```python
from build123d import *

# Parameters (mm, degrees)
ESQUISSE6_W                  = 10
ESQUISSE6_H                  = 1
ENL_V_MAT_EXTRU_3_DEPTH      = 4
ENL_V_MAT_EXTRU_3_DEPTH_BACK = 4


with BuildPart() as part:
    # Esquisse1 → R_volution5 (revolve)
    with BuildSketch(Plane.XY):
        Polygon((-18.5, 7.5), (44, 7.5), (45, 6.5), (45, 0), (-13.190313779, 0), (-15.499848989, 4.000151011), (-32.499848989, 4.000151011), (-32.499848989, 9.000151011), (-31.5, 10), (-18.5, 10), align=None)
    revolve(axis=Axis((-1000, 0, 0), (1, 0, 0)))

    # Esquisse5 → Enl_vement de mati_re-R_volution1 (revolve, cut)
    with BuildSketch(Plane.XY):
        Polygon((-29, 10), (-29, 3), (-27.75, 1.75), (-25, 1.75), (-25, 10), align=None)
    revolve(axis=Axis((-25, 1.75, 0), (0, 1, 0)), mode=Mode.SUBTRACT)

    # Esquisse6 → Enl_v. mat.-Extru.3 (cut, two sides)
    with BuildSketch(Plane.XY) as enl_v_mat_extru_3_sk:
        with Locations((30.5, 7)):
            Rectangle(ESQUISSE6_W, ESQUISSE6_H)
    extrude(amount=ENL_V_MAT_EXTRU_3_DEPTH, mode=Mode.SUBTRACT)
    extrude(enl_v_mat_extru_3_sk.sketch, amount=-ENL_V_MAT_EXTRU_3_DEPTH_BACK, mode=Mode.SUBTRACT)


solid = part.part
```
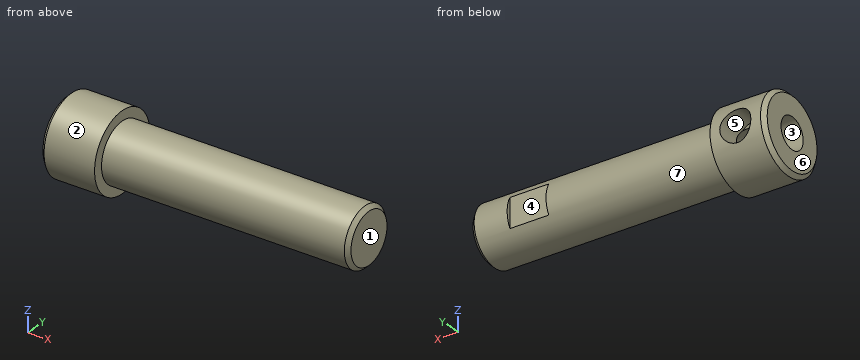
Check sheet for the modelled part. Datum: model origin and axes. Units: mm. Face numbers are marked on the shaded views. A direction names the side the tool comes from. Round coordinates to 2 decimals unless told otherwise and drop trailing zeros. Order: outer loops, then holes, each group sorted by start corner. A loop starts at its lowest first (then second) coordinate and runs counter-clockwise, first axis right, second up. Notation, with made-up numbers: (-23.75, 3.5) - (27.25, 3.5) arc R37 cw to (27.25, 42.5) - close; hole circle Ø3 at (88, -5). An arc over 180 degrees is marked (long way). Write item = value, one per line.
Q1. Tool access check on the marked faces 4, 5, 6 and 7. Record the directions out of +Z, -Z, +X, -X, +Y, -Y that give a thin tool (end or side, any length) a straight path to the whole face; none if there is none.
Computed:
face_4 = +Z, -Z, +Y
face_5 = +Y
face_6 = +Z, -Z, -X, +Y, -Y
face_7 = +X
Q2. Draft check along Z on the marked faces 1, 2 and 3. Enter one of: pulls with the +Z half, pulls with the -Z half, needs draft (parallel to the pull), parting line crosses it, or undercut.
Computed:
face_1 = needs draft
face_2 = parting line crosses it
face_3 = undercut
Q3. Thickness scan on line 1 along X through (y, z) = (8, 0); line 2 along X through (y, z) = (5.25, 7.25); line 3 along Z through (x, y) = (-25, 6.5). Record the ranges inside material, lowest first.
Computed:
line_1 = -32.5 to -29, -21 to -18.5
line_2 = -32.5 to -18.5
line_3 = -7.6 to -4, 4 to 7.6
Q4. Go/stop test with flat-tipped pins: pin 1 (2 mm diameter, centred on x = -9.5, z = -3, fed in from +Y); pin 2 (3 mm diameter, centred on x = -9, z = -1.5, fed in from +Y); pin 3 (6.5 mm diameter, centred on x = -25, z = 0, fed in from +Y). Record where each tip stops, or that it passes through.
Computed:
pin_1 = 7.23
pin_2 = 7.5
pin_3 = -2.33
Q5. Section check C-C (x = -7.5). Record the boundary of the cut face in (y, z), and give its area (3 significant figures).
Computed:
outline = circle Ø15 at (0, 0)
area = 177 mm^2
Q6. Section check B-B (x = 34). Record the boundary of the cut face in (y, z).
Computed:
outline = (6.5, -3.74) - (6.5, 3.74) arc R7.5 ccw (long way) to start
Q7. Section check A-A (x = -19.5). Record the boundary of the cut face in (y, z).
Computed:
outline = circle Ø20 at (0, 0); hole circle Ø8 at (0, 0)
